from build123d import *

# Parameters (mm, degrees)
CROQUIS1_W              = 8
CROQUIS1_H              = 13
SALIENTE_EXTRUIR1_DEPTH = 15
CROQUIS3_R              = 11
CORTAR_EXTRUIR1_DEPTH   = 15
CROQUIS4_R              = 2.5
CORTAR_EXTRUIR2_DEPTH   = 30
REDONDEO1_R             = 10
CROQUIS5_R              = 2.5
CORTAR_EXTRUIR3_DEPTH   = 2
BOSS_EXTRUDE1_REACH     = 44.403
SKETCH2_R               = 2.5
CUT_EXTRUDE1_DEPTH      = 3
BOSS_EXTRUDE2_START     = -14
SKETCH3_R               = 11
SKETCH3_R_2             = 4
BOSS_EXTRUDE2_DEPTH     = 14
SKETCH4_R               = 2.5
BOSS_EXTRUDE4_DEPTH     = 2


with BuildPart() as part:
    # Croquis1 → Saliente-Extruir1 (new, symmetric)
    with BuildSketch(Plane.XY):
        Polygon((-15, -2), (-7, -2), (-7, -15), (-15, -15), (-15, -17), (-8, -17), (-8, -33), (-6, -33), (-6, -17), (6, -17), (6, -33), (8, -33), (8, -17), (15, -17), (15, -15), (7, -15), (7, -2), (15, -2), (15, 2), (7, 2), (7, 15), (15, 15), (15, 17), (-15, 17), (-15, 15), (-7, 15), (-7, 2), (-15, 2), align=None)
        with Locations((0, 8.5)):
            Rectangle(CROQUIS1_W, CROQUIS1_H, mode=Mode.SUBTRACT)
        with Locations((0, -8.5)):
            Rectangle(CROQUIS1_W, CROQUIS1_H, mode=Mode.SUBTRACT)
    extrude(amount=SALIENTE_EXTRUIR1_DEPTH, both=True)

    # Croquis3 → Cortar-Extruir1 (cut, symmetric)
    with BuildSketch(Plane(origin=(0, 0, 0), x_dir=(0, 0, -1), z_dir=(1, 0, 0))):
        with Locations(Location((0, 0, 0), (0, 0, 10.475681696))):
            Circle(CROQUIS3_R)
    extrude(amount=CORTAR_EXTRUIR1_DEPTH, both=True, mode=Mode.SUBTRACT)

    # Croquis4 → Cortar-Extruir2 (cut)
    with BuildSketch(Plane(origin=(8, 0, 0), x_dir=(0, 0, -1), z_dir=(1, 0, 0))):
        with Locations(Location((-8, -25, 0), (0, 0, 90))):
            Circle(CROQUIS4_R)
        with Locations(Location((8, -25, 0), (0, 0, 90))):
            Circle(CROQUIS4_R)
    extrude(amount=-CORTAR_EXTRUIR2_DEPTH, mode=Mode.SUBTRACT)

    # Redondeo1
    redondeo1_edges = [part.edges().sort_by_distance(p)[0] for p in [
        (7, -33, -15),
        (-7, -33, -15),
        (-7, -33, 15),
        (7, -33, 15),
    ]]
    fillet(redondeo1_edges, radius=REDONDEO1_R)

    # Croquis5 → Cortar-Extruir3 (cut)
    with BuildSketch(Plane(origin=(0, 17, 0), x_dir=(1, 0, 0), z_dir=(0, 1, 0))):
        with Locations(Location((-11, 0, 0), (0, 0, 270))):
            Circle(CROQUIS5_R)
        with Locations(Location((11, 0, 0), (0, 0, 270))):
            Circle(CROQUIS5_R)
    extrude(amount=-CORTAR_EXTRUIR3_DEPTH, mode=Mode.SUBTRACT)

    # Boss-Extrude1: up to this face of the body (flat: up to its plane)
    boss_extrude1_end = Plane(part.part.faces().sort_by_distance((15, 0, 12.969177885))[0])
    # Sketch1 → Boss-Extrude1 (add, up to the picked face)
    with BuildSketch(Plane(origin=(7, 0, 0), x_dir=(0, 0, -1), z_dir=(1, 0, 0)), mode=Mode.PRIVATE) as boss_extrude1_sk1:
        with BuildLine():
            Line((-2, 15), (2, 15))
            Line((2, 15), (2, 10.816653826))
            ThreePointArc((2, 10.816653826), (0, 11), (-2, 10.816653826))
            Line((-2, 10.816653826), (-2, 15))
        make_face()
    boss_extrude1_tool1 = split(extrude(boss_extrude1_sk1.sketch, amount=BOSS_EXTRUDE1_REACH, mode=Mode.PRIVATE), bisect_by=boss_extrude1_end, keep=Keep.BOTH, mode=Mode.PRIVATE)
    boss_extrude1 = boss_extrude1_tool1.solids().sort_by(Axis((7, 12.969178, 0), (1, 0, 0)))[0]
    add(boss_extrude1)

    # Mirror1: Boss-Extrude1 across plane
    add(boss_extrude1.mirror(Plane.ZX))

    # Sketch2 → Cut-Extrude1 (cut)
    with BuildSketch(Plane(origin=(7, 0, 0), x_dir=(0, 0, -1), z_dir=(1, 0, 0))):
        with Locations(Location((-10.7, 10.7, 0), (0, 0, 90))):
            Circle(SKETCH2_R)
        with Locations(Location((10.7, -10.7, 0), (0, 0, 90))):
            Circle(SKETCH2_R)
    extrude(amount=-CUT_EXTRUDE1_DEPTH, mode=Mode.SUBTRACT)

    # Sketch3 → Boss-Extrude2 (add)
    with BuildSketch(Plane.ZY.offset(7).offset(BOSS_EXTRUDE2_START)):
        Circle(SKETCH3_R)
        with Locations(Location((0, 0, 0), (0, 0, 270))):
            Circle(SKETCH3_R_2, mode=Mode.SUBTRACT)
    boss_extrude2 = extrude(amount=BOSS_EXTRUDE2_DEPTH)

    # Mirror2: Boss-Extrude2 across plane
    add(boss_extrude2.mirror(Plane(origin=(0, 0, 0), x_dir=(0, 0, 1), z_dir=(1, 0, 0))))

    # Sketch4 → Boss-Extrude4 (add)
    with BuildSketch(Plane(origin=(0, 17, 0), x_dir=(1, 0, 0), z_dir=(0, 1, 0))):
        with Locations((11, 0)):
            Circle(SKETCH4_R)
    extrude(amount=-BOSS_EXTRUDE4_DEPTH)


solid = part.part
Work out the finished part from the listing and answer in its coordinate system (mm). A direction names the side the tool comes from. Coordinates: 2 decimals unless noted, no trailing zeros. Write each loop counter-clockwise with the first axis right and the second up, starting at its lowest first coordinate (ties: lowest second). Pieces come first, ordered by that corner, then holes.
1. The part is cut by section D-D, the plane z = 0. State how many separate pieces and enclosed holes the cut face has, and give its area (3 significant figures).
Results list:
separate pieces: 3
enclosed holes: 2
area: 482 mm2
2. For a pull along Y with two mould halves and no side action, classify faces 4 (the flat face through (-8, -25, 0)), 5 (the cylindrical face through (7.01, -29.99, -12.15)), 6 (the flat face through (-11, 2, 13)) as +Y half, -Y half, draft (parallel to the pull), parting line (faces both ways), or undercut.
Results list:
face 4: draft
face 5: -Y half
face 6: undercut
3. The part is cut by section C-C, the plane x = 12.5. Write down the section's boundary in (y, z).
Results list:
outline: (-17, -15) - (-15, -15) - (-15, -2) - (-10.82, -2) arc R11 cw to (-10.82, 2) - (-15, 2) - (-15, 15) - (-17, 15) - close; (-2, -15) - (2, -15) - (2, -10.82) arc R11 cw to (-2, -10.82) - close; (-2, 10.82) arc R11 cw to (2, 10.82) - (2, 15) - (-2, 15) - close; (10.82, -2) - (15, -2) - (15, -15) - (17, -15) - (17, 15) - (15, 15) - (15, 2) - (10.82, 2) arc R11 cw to start
4. The part is cut by section B-B, the plane y = 0. Write down the section's boundary in (x, z), and give its area (3 significant figures).
Results list:
outline: (-15, -15) - (15, -15) - (15, -11) - (7, -11) - (7, -4) - (-7, -4) - (-7, -11) - (-15, -11) - close; (-15, 11) - (-7, 11) - (-7, 4) - (7, 4) - (7, 11) - (15, 11) - (15, 15) - (-15, 15) - close
area: 436 mm2
5. Consider line 1 along Y through (x, z) = (-3.25, 12); line 2 along Y through (x, z) = (-2.5, 9); line 3 along Z through (x, y) = (1.5, 0). Determine where each line is inside the solid, lowest interval first.
Results list:
line 1: y = -17 to -15, -2 to 2, 15 to 17
line 2: y = -17 to -15, -6.32 to 6.32, 15 to 17
line 3: z = -15 to -4, 4 to 15
6. For faces 1 (the flat face through (11, 2, -13)), 2 (the cylindrical face through (11, 0, 11)), 3 (the cylindrical face through (0, 11, 0)), determine the directions among +Z, -Z, +X, -X, +Y, -Y from which every point of the face is accessible in a straight line to the end or side of a thin tool.
Results list:
face 1: +Z, -Z, +X
face 2: +X
face 3: none
7. The part is cut by section A-A, the plane x = 0. Write down the section's boundary in (y, z), and give its area (3 significant figures).
Results list:
outline: (-17, -15) - (-15, -15) - (-15, 15) - (-17, 15) - close; (-2, -15) - (2, -15) - (2, -10.82) arc R11 ccw to (2, 10.82) - (2, 15) - (-2, 15) - (-2, 10.82) arc R11 ccw to (-2, -10.82) - close; (15, -15) - (17, -15) - (17, 15) - (15, 15) - close; hole circle Ø8 at (0, 0)
area: 482 mm2
8. Flat-ended cylindrical pins translate along their axes: pin 1 (15 mm diameter, centred on y = 1, z = -1.5, fed in from -X); pin 2 (4 mm diameter, centred on y = -25, z = 8, fed in from +X); pin 3 (2.5 mm diameter, centred on x = 9, z = 8.5, fed in from -Y); pin 4 (4.5 mm diameter, centred on x = -1, z = -12, fed in from -Y). Find the tip coordinate at first contact, or state that the pin passes through.
Results list:
pin 1: stops at x = -7
pin 2: passes through
pin 3: stops at y = -32.61
pin 4: stops at y = -17
